Could you check a few things on this model? Use its own coordinates, in mm. A direction names the side the tool comes from. Round coordinates to 2 decimals unless told otherwise and drop trailing zeros. Return JSON: item names as keys, results as strings. Group by question number.
```python
from build123d import *

# Parameters (mm, degrees)
F1_DEPTH = 6.35
F4_D     = 3.571875
F4_DEPTH = 12.7
F4_TIP   = 1.0730995118
F5_D     = 3.571875
F5_DEPTH = 12.7
F5_TIP   = 1.0730995118


with BuildPart() as f1:
    # F0 (on Right) → F1 (new body)
    with BuildSketch(Plane.YZ):
        Polygon((0, 41.275), (0, 0), (76.2, 0), (41.5661627232, 41.275), align=None)
    extrude(amount=F1_DEPTH)

    # F4
    with Locations(Plane.XZ):
        with Locations((3.175, 30.95625), (3.175, 10.31875), (3.175, 20.6375)):
            Hole(F4_D / 2, depth=F4_DEPTH)
            with Locations((0, 0, -(F4_DEPTH + F4_TIP / 2))):  # 118° drill point
                Cone(0, F4_D / 2, F4_TIP, mode=Mode.SUBTRACT)

    # F5
    with Locations(Plane(origin=(0, 44.7159955691, 37.5211753898), x_dir=(-1, 0, 0), z_dir=(0, 0.7660444431, 0.6427876097))):
        with Locations((-3.175, -8.5699014577), (-3.175, -22.0400729245), (-3.175, -35.5102443913)):
            Hole(F5_D / 2, depth=F5_DEPTH)
            with Locations((0, 0, -(F5_DEPTH + F5_TIP / 2))):  # 118° drill point
                Cone(0, F5_D / 2, F5_TIP, mode=Mode.SUBTRACT)


solid = f1.part
```
1. I need wall thicknesses on probe 1 along Z at (x, y) = (4.5, 3) (3 decimals); probe 2 along Y at (x, z) = (3.75, 24.5); probe 3 along Y at (x, z) = (1.75, 26.5). Which ranges of each line are inside material? Lowest first, please.
2. We'd pull the mould along X, two halves only. Please class faces 1 (the face through (3.242, 57.328, 1.353)), 2 (the face through (0, 29, 21)), 3 (the face through (6.35, 29, 21)): +X half, -X half, draft (parallel to the pull), parting line (faces both ways), or undercut.
3. I'm going to push flat-ended pins straight in: pin 1 Ø2 at (x, z) = (1, 35) entering from +Y; pin 2 Ø1.5 at (x, y) = (4.5, 64.5) entering from +Z; pin 3 Ø2 at (x, z) = (4.5, 24) entering from +Y. Where does each tip first touch, or does it pass through?
4. On a 3-axis mill with a long thin cutter (end or side, diameter ignored), from which of +Z, -Z, +X, -X, +Y, -Y can I reach the whole of each face in a straight line? I mean faces 4 (the face through (5.2, 0, 20.9)), 5 (the face through (3.24, 40.01, 21.99)), 6 (the face through (3.562, 6.439, 8.575)). Say none if no direction works.
Geometry results:
{
 "1": {"probe 1": "0 to 9.121, 11.516 to 19.44, 21.835 to 29.759, 32.154 to 41.275", "probe 2": "0 to 39.9, 45.16 to 55.64", "probe 3": "0 to 43.24, 46.59 to 53.96"},
 "2": {"face 1": "undercut", "face 2": "-X half", "face 3": "+X half"},
 "3": {"pin 1": "y = 47.67", "pin 2": "z = 14.84", "pin 3": "y = 56.9"},
 "4": {"face 4": "+Z, -Z, +X, -X, -Y", "face 5": "none", "face 6": "-Y"}
}
